Input: part model. Units: mm. Frame: model coordinates. Give positions to 0.01 mm unless a question says otherwise; leave off trailing zeros. Loops run counter-clockwise (first coordinate to the right, second up) from the corner with the lowest first, then second, coordinate; pieces in that order, holes last. Notation, with made-up numbers: (65.25, 9) - (90.25, 9) arc R10 cw to (90.25, 14) - close; hole circle Ø1 at (-19.5, 38). An arc over 180 degrees is marked (long way). Answer as a JSON object with one key per item and string values. Group by question number.
(1) Pin query (flat end, axial travel): P1, Ø10, axis at x = 40.5, z = -11.5, coming from the +Y side; P2, Ø3, axis at x = 25, y = -5.5, coming from the +Z side. Return the tip coordinate at first contact, or that it passes through.
(2) Material intervals for L1, parallel to Z at x = 19, y = 19.5; L2, parallel to X at y = -18, z = -15.5; L3, parallel to X at y = -18.5, z = -7, sorted ascending.
(3) Section query C-C (z = -5). Return loops of the section in (x, y).
(4) Section query B-B (x = 44). Return loops of the section in (y, z).
(5) Section query A-A (y = -1). Return loops of the section in (x, z), plus the area to 3 significant figures.
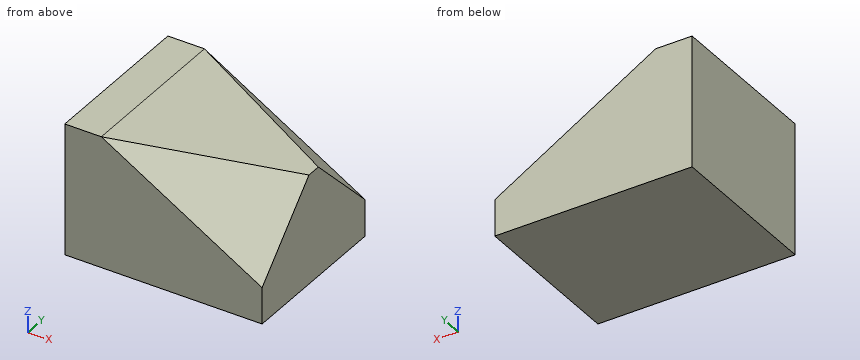
Autodesk Inventor part; units mm, degrees
ref_plane "工作平面1" through (10, 22, 0) normal (-0.3855, -0.6524, -0.6524) x (0.8609, 0, -0.5087)
ref_plane "YZ Plane" through (0, 0, 0) normal (1, 0, 0) x (0, 1, 0)
ref_plane "XZ Plane" through (0, 0, 0) normal (0, 1, 0) x (-1, 0, 0)
sketch "草圖1" plane through (0, 0, 0) normal (0, 1, 0) x (-1, 0, 0)
  line L0 (0, 0) -> (-54, 0)
  line L1 (-54, 0) -> (-54, -36)
  line L2 (-54, -36) -> (0, -36)
  line L3 (0, -36) -> (0, 0)
  dimension "d0" = 54
  dimension "d1" = 36
extrude "擠出1" add sketch "草圖1" along normal mid plane 44
sketch "草圖2" plane through (0, 22, 0) normal (0, 1, 0) x (1, 0, 0)
  line L0 (0, 0) -> (54, 0)
  line L1 (10, 0) -> (54, 6)
  line L2 (54, 0) -> (54, 36)
  dimension "d4" = 10
  dimension "d5" = 30
extrude "擠出2" cut sketch "草圖2" against normal blind 60
sketch "草圖3" plane through (54, -22, -36) normal (1, 0, 0) x (0, 0, -1)
  line L0 (-30, 24) -> (-10, 44)
  line L1 (0, 44) -> (-36, 44)
  line L2 (-30, 44) -> (-30, 0)
  point P0 (-36, 22)
  point P1 (-30, 2)
  dimension "d8" = 20
  dimension "d9" = 20
ref_plane "工作平面1" through (10, 22, 0) normal (-0.3855, -0.6524, -0.6524) x (0.8609, 0, -0.5087)
sketch "草圖4" plane through (10, 22, 0) normal (-0.3855, -0.6524, -0.6524) x (0.8609, 0, -0.5087)
  line L0 (-15.1543, -12.3218) -> (93.717, -12.3218)
  line L1 (93.717, -12.3218) -> (93.717, 28.8166)
  line L2 (93.717, 28.8166) -> (-15.1543, 28.8166)
  line L3 (-15.1543, 28.8166) -> (-15.1543, -12.3218)
  point P0 (-8.6093, 13.3533)
extrude "擠出3" cut sketch "草圖4" against normal blind 40
mirror "鏡射1" about plane through (0, 0, 0) normal (0, 1, 0) of "擠出3"
properties part number "46"
Recorded:
{
 "1": {"P1": "stops at y = 21.28", "P2": "stops at z = -1.84"},
 "2": {"L1": "z = -36 to -2.82", "L2": "x = 0 to 43", "L3": "x = 0 to 27.76"},
 "3": {"outline": "(0, -22) - (18.46, -22) - (46.67, -5.33) - (46.67, 5.33) - (18.46, 22) - (0, 22) - close"},
 "4": {"outline": "(-22, -36) - (22, -36) - (22, -20.09) - (6.54, -4.64) - (-6.54, -4.64) - (-22, -20.09) - close"},
 "5": {"outline": "(0, -36) - (54, -36) - (54, -6) - (10, 0) - (0, 0) - close", "area": "1,810 mm^2"}
}
